Source: CAD feature listing. Evaluate the final solid. Frame: model axes, mm. Face numbers are marked on the shaded views. A direction names the side the tool comes from. Give positions to 0.01 mm unless a question says otherwise; leave off trailing zeros. Loops run counter-clockwise (first coordinate to the right, second up) from the corner with the lowest first, then second, coordinate; pieces in that order, holes last.
from build123d import *

# Parameters (mm, degrees)
F0_W           = 7
F0_H           = 9
F0_H_2         = 13
F0_W_2         = 22
F0_H_3         = 9.5
F1_DEPTH       = 10
F2_D           = 4.2
F3_SIZE        = 5
F4_D           = 5.5
F4_CBORE_D     = 9.75
F4_CBORE_DEPTH = 5


with BuildPart() as f1:
    # F0 (on Top) → F1 (new body)
    with BuildSketch(Plane.XY):
        with Locations((45.9692735374, -36.8180999458)):
            Rectangle(F0_W, F0_H)
        with Locations((45.9692735374, -16.3180999458)):
            Rectangle(F0_W, F0_H_2)
        with Locations((45.9692735374, 4.1819000542)):
            Rectangle(F0_W, F0_H)
        with Locations((24.4692735374, 4.1819000542)):
            Rectangle(F0_W_2, F0_H)
        with Locations((2.9692735374, 4.1819000542)):
            Rectangle(F0_W, F0_H)
        with Locations((2.9692735374, -16.3180999458)):
            Rectangle(F0_W, F0_H_2)
        with Locations((24.4692735374, -16.3180999458)):
            Rectangle(F0_W_2, F0_H_2)
        with Locations((24.4692735374, -36.8180999458)):
            Rectangle(F0_W_2, F0_H)
        with Locations((2.9692735374, -36.8180999458)):
            Rectangle(F0_W, F0_H)
        with Locations((2.9692735374, -5.0680999458)):
            Rectangle(F0_W, F0_H_3)
        with Locations((9.9692735374, -5.0680999458)):
            Rectangle(F0_W, F0_H_3)
        with Locations((9.9692735374, 4.1819000542)):
            Rectangle(F0_W, F0_H)
        with Locations((24.4692735374, -5.0680999458)):
            Rectangle(F0_W_2, F0_H_3)
        with Locations((38.9692735374, -5.0680999458)):
            Rectangle(F0_W, F0_H_3)
        with Locations((38.9692735374, 4.1819000542)):
            Rectangle(F0_W, F0_H)
        with Locations((45.9692735374, -5.0680999458)):
            Rectangle(F0_W, F0_H_3)
        with Locations((38.9692735374, -16.3180999458)):
            Rectangle(F0_W, F0_H_2)
        with Locations((9.9692735374, -16.3180999458)):
            Rectangle(F0_W, F0_H_2)
        with Locations((2.9692735374, -27.5680999458)):
            Rectangle(F0_W, F0_H_3)
        with Locations((9.9692735374, -27.5680999458)):
            Rectangle(F0_W, F0_H_3)
        with Locations((24.4692735374, -27.5680999458)):
            Rectangle(F0_W_2, F0_H_3)
        with Locations((38.9692735374, -27.5680999458)):
            Rectangle(F0_W, F0_H_3)
        with Locations((45.9692735374, -27.5680999458)):
            Rectangle(F0_W, F0_H_3)
        with Locations((9.9692735374, -36.8180999458)):
            Rectangle(F0_W, F0_H)
        with Locations((38.9692735374, -36.8180999458)):
            Rectangle(F0_W, F0_H)
    extrude(amount=F1_DEPTH)

    # F2 (through all)
    with Locations(Plane(origin=(0, 0, 0), x_dir=(1, 0, 0), z_dir=(0, 0, -1))):
        with Locations((13.4692735374, 9.8180999458), (35.4692735374, 9.8180999458), (35.4692735374, 22.8180999458), (13.4692735374, 22.8180999458)):
            Hole(F2_D / 2)

    # F3
    f3_edges = [f1.edges().sort_by_distance(p)[0] for p in [
        (49.469274, 8.6819, 5),
        (49.469274, -41.3181, 5),
        (-0.530726, -41.3181, 5),
        (-0.530726, 8.6819, 5),
    ]]
    chamfer(f3_edges, length=F3_SIZE)

    # F4 (through all)
    with Locations(Plane(origin=(0, 0, 0), x_dir=(1, 0, 0), z_dir=(0, 0, -1))):
        with Locations((6.4692735374, 0.3180999458), (42.4692735374, 32.3180999458)):
            CounterBoreHole(F4_D / 2, F4_CBORE_D / 2, F4_CBORE_DEPTH)


with BuildPart() as f5_1:
    # F5: instance of F1
    add(f1.part.mirror(Plane.XY))


solid = f5_1.part
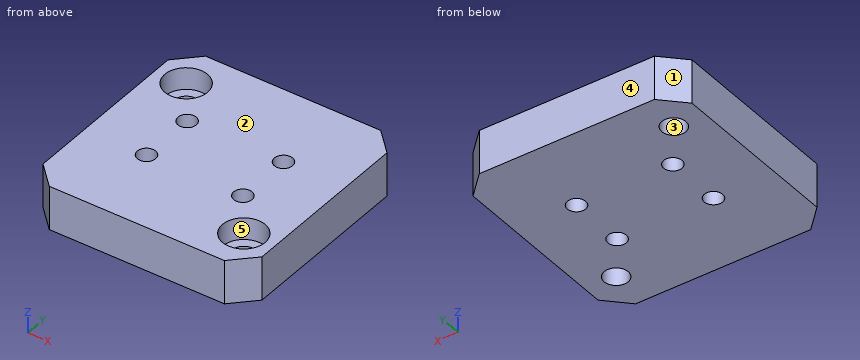
1) Reachability of the marked faces 4 and 5 from +Z, -Z, +X, -X, +Y, -Y: full face, straight path, thin tool, end or side. Return the list, or none.
Checks:
face 4: +Z, -Z, +X, -X, +Y
face 5: +Z
2) Pull-direction query (X, two-part tool) for the marked faces 1, 2 and 3; classes: released by +X, released by -X, zero draft, split by the parting line, or undercut.
Checks:
face 1: released by -X
face 2: zero draft
face 3: undercut
3) Contact query for flat-ended pins moving along their axis: P1, Ø7, axis at x = 42.47, y = -32.32, coming from the +Z side; P2, Ø3.5, axis at x = 13.47, y = -22.82, coming from the -Z side. Output: stop coordinate, or through.
Checks:
P1: stops at z = -5
P2: passes through
4) Cut plane C-C (x = 36.5). Return loops of the section in (y, z), and give its area (3 significant figures).
Checks:
outline: (-41.32, -10) - (-24.65, -10) - (-24.65, 0) - (-41.32, 0) - close; (-20.99, -10) - (-11.65, -10) - (-11.65, 0) - (-20.99, 0) - close; (-7.99, -10) - (8.68, -10) - (8.68, 0) - (-7.99, 0) - close
area: 427 mm2
5) Ray query, probe 1 along X at (y, z) = (-32.5, -9.25); probe 2 along X at (y, z) = (-11, -7.5); probe 3 along Y at (x, z) = (14, -3.5). Return the intervals inside material, ascending.
Checks:
probe 1: x = -0.53 to 39.73, 45.21 to 49.47
probe 2: x = -0.53 to 11.73, 15.21 to 33.73, 37.21 to 49.47
probe 3: y = -41.32 to -24.85, -20.79 to -11.85, -7.79 to 8.68
6) Cut plane D-D (z = -2). Return loops of the section in (x, y) (3 decimals).
Checks:
outline: (-0.531, -36.318) - (4.469, -41.318) - (44.469, -41.318) - (49.469, -36.318) - (49.469, 3.682) - (44.469, 8.682) - (4.469, 8.682) - (-0.531, 3.682) - close; hole circle Ø9.75 at (6.469, -0.318); hole circle Ø4.2 at (13.469, -22.818); hole circle Ø4.2 at (13.469, -9.818); hole circle Ø4.2 at (35.469, -22.818); hole circle Ø4.2 at (35.469, -9.818); hole circle Ø9.75 at (42.469, -32.318)
7) Cut plane B-B (y = -24). Return loops of the section in (x, z).
Checks:
outline: (-0.53, -10) - (11.73, -10) - (11.73, 0) - (-0.53, 0) - close; (15.21, -10) - (33.73, -10) - (33.73, 0) - (15.21, 0) - close; (37.21, -10) - (49.47, -10) - (49.47, 0) - (37.21, 0) - close
8) Cut plane A-A (z = -6.25). Return loops of the section in (x, y).
Checks:
outline: (-0.53, -36.32) - (4.47, -41.32) - (44.47, -41.32) - (49.47, -36.32) - (49.47, 3.68) - (44.47, 8.68) - (4.47, 8.68) - (-0.53, 3.68) - close; hole circle Ø5.5 at (6.47, -0.32); hole circle Ø4.2 at (13.47, -22.82); hole circle Ø4.2 at (13.47, -9.82); hole circle Ø4.2 at (35.47, -22.82); hole circle Ø4.2 at (35.47, -9.82); hole circle Ø5.5 at (42.47, -32.32)
